Input: part model. Units: mm. Frame: model coordinates. A direction names the side the tool comes from. Coordinates: 2 decimals unless noted, no trailing zeros. Loops run counter-clockwise (first coordinate to the right, second up) from the corner with the lowest first, then second, coordinate; pieces in that order, holes last. Notation, with made-up numbers: M -28.5,55 L -20.5,55 A19 cw -20.5,83 Z; hole C -31.5,56.25 d6. An arc over 180 degrees is marked long. Use a Markdown table: item, result. Add a question column.
1. Draft query along X for faces 1 (the cylindrical face through (30, 9, 44)), 2 (the flat face through (0, 4, 13)), 3 (the flat face through (16, -2, 31)), 4 (the flat face through (34, 4, 31)). Return one class per face: +X half, -X half, draft (parallel to the pull), parting line (faces both ways), or undercut.
2. Section B-B on z = 13.5. Output: boundary loops of the cut face in (x, y).
3. Section C-C on x = 2.5. Output: boundary loops of the cut face in (y, z).
4. Pin query (flat end, axial travel): pin 1 (4 mm diameter, centred on x = 3, y = 2.5, fed in from -Z); pin 2 (10 mm diameter, centred on x = 12, z = 43.5, fed in from +Y); pin 3 (2.5 mm diameter, centred on y = 2, z = 44.5, fed in from -X). Return the tip coordinate at first contact, or that it passes through.
5. Set-up query: faces 5 (the flat face through (8, 9, 56)), 6 (the flat face through (32, 4, 30)), 7 (the flat face through (-1, 4, 26)). Return all of +Z, -Z, +X, -X, +Y, -Y with unobstructed straight access to the full face (end or side cutting, diameter ignored); none if empty.
6. Section D-D on z = 44. Output: boundary loops of the cut face in (x, y).
7. Line query: L1, parallel to X at y = 3, z = 11; L2, parallel to Y at x = 25, z = 56.5; L3, parallel to Z at x = 18.5, y = 9. Output: solid intervals per line, ascending. Write a range as [from, to].
8. Section A-A on y = 6.75. Output: boundary loops of the cut face in (x, z).
Autodesk Inventor part; units mm, degrees
ref_plane "YZ Plane" through (0, 0, 0) normal (1, 0, 0) x (0, 1, 0)
ref_plane "XZ Plane" through (0, 0, 0) normal (0, 1, 0) x (-1, 0, 0)
ref_plane "XY Plane" through (0, 0, 0) normal (0, 0, 1) x (1, 0, 0)
sketch "Sketch1" plane through (0, 0, 0) normal (0, 0, 1) x (1, 0, 0)
  line L0 (0, 0) -> (32, 0)
  line L1 (32, 0) -> (32, 8)
  line L2 (32, 8) -> (0, 8)
  line L3 (0, 8) -> (0, 0)
  line L4 (-2, 10) -> (34, 10)
  line L5 (34, 10) -> (34, -2)
  line L6 (34, -2) -> (-2, -2)
  line L7 (-2, -2) -> (-2, 10)
  dimension "d0" = 32
  dimension "d1" = 8
  dimension "d2" = 2
  dimension "d3" = 2
  dimension "d4" = 2
  dimension "d5" = 2
extrude "Extrusion1" add sketch "Sketch1" along normal blind 60
sketch "Sketch3" plane through (0, 0, 60) normal (0, 0, 1) x (1, 0, 0)
  line L0 (34, 10) -> (-2, 10)
  line L1 (-2, -2) -> (34, -2)
  line L2 (34, -2) -> (34, 10)
  line L3 (34, 10) -> (-2, 10)
  line L4 (-2, 10) -> (-2, -2)
  line L5 (0, 0) -> (0, 8)
  line L6 (0, 8) -> (32, 8)
  line L7 (32, 8) -> (32, 0)
  line L8 (32, 0) -> (0, 0)
  point P0 (-2, 10)
extrude "Extrusion2" add sketch "Sketch3" along normal blind 3 contours L2 L1 L4 L0 | L5 L6 L7 L8
sketch "Sketch4" plane through (-2, -2, 0) normal (-1, 0, 0) x (0, 0, 1)
  line L0 (26, 2) -> (60, 2)
  line L1 (60, 2) -> (60, 10)
  line L2 (60, 10) -> (26, 10)
  line L3 (26, 10) -> (26, 2)
  line L4 (0, 12) -> (63, 12)
  line L5 (63, 12) -> (63, 0)
  point P0 (0, 2)
  point P1 (43, 10)
  dimension "d11" = 8
  dimension "d12" = 2
  dimension "d13" = 34
  dimension "d16" = 3
extrude "Extrusion3" cut sketch "Sketch4" against normal blind 3
sketch "Sketch2" plane through (-2, 10, 0) normal (0, 1, 0) x (1, 0, 0)
  line L0 (20, -44) -> (-20, -44) construction
  line L1 (20, -56) -> (-20, -56)
  line L2 (-20, -32) -> (20, -32)
  arc A0 (20, -56) -> (20, -32) centre (20, -44) ccw
  arc A1 (-20, -32) -> (-20, -56) centre (-20, -44) ccw
  line L3 (0, 0) -> (0, -63)
  point P0 (2, 0)
  point P1 (0, -44)
  point P2 (0, -26)
  point P3 (0, -60)
  point P4 (0, -32)
  point P5 (0, -56)
  dimension "d8" = 24
  dimension "d17" = 18
  dimension "d18" = 20
  dimension "d19" = 40
extrude "Extrusion4" cut sketch "Sketch2" against normal blind 3 contours L1 L3 L2 A0
properties part number "prototype2_2"
Answers below:
| question | item | result |
|---|---|---|
| 1 | face 1 | -X half |
| 1 | face 2 | undercut |
| 1 | face 3 | draft |
| 1 | face 4 | +X half |
| 2 | outline | M -2,-2 L 34,-2 L 34,10 L -2,10 Z; hole M 0,0 L 32,0 L 32,8 L 0,8 Z |
| 3 | outline | M -2,0 L 0,0 L 0,60 L 8,60 L 8,56 L 10,56 L 10,63 L -2,63 Z; M 8,0 L 10,0 L 10,32 L 8,32 Z |
| 4 | pin 1 | stops at z = 60 |
| 4 | pin 2 | stops at y = 0 |
| 4 | pin 3 | stops at x = 32 |
| 5 | face 5 | -X, +Y |
| 5 | face 6 | -Z |
| 5 | face 7 | -X |
| 6 | outline | M -2,-2 L 34,-2 L 34,10 L 30,10 L 30,8 L 32,8 L 32,0 L -2,0 Z |
| 7 | L1 | x = [-2, 0], [32, 34] |
| 7 | L2 | y = [-2, 0], [8, 10] |
| 7 | L3 | z = [0, 32.01], [55.99, 63] |
| 8 | outline | M -2,0 L 0,0 L 0,26 L -2,26 Z; M -2,60 L 32,60 L 32,0 L 34,0 L 34,63 L -2,63 Z |
